from build123d import *

# Parameters (mm, degrees)
CROQUIS1_R                   = 2.5000000000000004
SALIENTE_EXTRUIR1_DEPTH      = 10
SALIENTE_EXTRUIR2_DEPTH      = 12
CROQUIS3_R                   = 1.5000000000000024
SALIENTE_EXTRUIR3_DEPTH      = 2
REDONDEO1_R                  = 2
CROQUIS4_R                   = 1.5000000000000024
CORTAR_EXTRUIR1_DEPTH        = 6
SALIENTE_EXTRUIR4_DEPTH      = 3.21644
SALIENTE_EXTRUIR4_DEPTH_BACK = 18.409513
CROQUIS6_R                   = 2.5
SALIENTE_EXTRUIR5_START      = -21.625954
SALIENTE_EXTRUIR5_DEPTH      = 21.625954


with BuildPart() as part:
    # Croquis1 → Saliente-Extruir1 (new body)
    with BuildSketch(Plane(origin=(0, 0, 0), x_dir=(1, 0, 0), z_dir=(0, 1, 0))):
        with BuildLine():
            Line((0, -4.5), (4.5, -4.5))
            Line((4.5, -4.5), (4.5, 0))
            Line((4.5, 0), (4.5, 4.5))
            Line((4.5, 4.5), (0, 4.5))
            ThreePointArc((0, 4.5), (-4.5, 5.5e-16), (0, -4.5))
        make_face()
        with Locations(Location((0, 0, 0), (0, 0, 270))):
            Circle(CROQUIS1_R, mode=Mode.SUBTRACT)
    extrude(amount=SALIENTE_EXTRUIR1_DEPTH)

    # Croquis2 → Saliente-Extruir2 (add)
    with BuildSketch(Plane(origin=(4.5, 0, 0), x_dir=(0, 0, -1), z_dir=(1, 0, 0))):
        Polygon((-4.5, 0), (-4.5, 1.7434467956210846), (4.5, 14.596778856299984), (4.5, 11.10988526505781), (-3.2792254112385364, 0), align=None)
    extrude(amount=SALIENTE_EXTRUIR2_DEPTH)

    # Croquis3 → Saliente-Extruir3 (add)
    with BuildSketch(Plane(origin=(0, 2.68788483311935, 3.838697366771722), x_dir=(1, 0, 0), z_dir=(0, 0.57357643635105, 0.819152044288989))):
        Polygon((4.5, 19.19256462345726), (16.5, 19.19256462345726), (16.500000000000004, -5.807435376542737), (4.500000000000008, -5.807435376542739), align=None)
        with Locations(Location((10.5, 14.692564623457262, 0), (0, 0, 270))):
            Circle(CROQUIS3_R, mode=Mode.SUBTRACT)
        with Locations((10.500000000000002, -1.307435376542739)):
            Circle(CROQUIS3_R, mode=Mode.SUBTRACT)
    extrude(amount=-SALIENTE_EXTRUIR3_DEPTH)

    # Redondeo1
    # the kernel refuses this fillet: 2 mm, written as the material it adds along each edge
    with BuildSketch(Plane(origin=(4.5, 14.095760221444946, -6.590732152613882), x_dir=(0, -0.5735764363510499, -0.8191520442889891), z_dir=(0, -0.8191520442889891, 0.5735764363510499))) as redondeo1_piece_1_section:
        with BuildLine():
            CenterArc((REDONDEO1_R, REDONDEO1_R), REDONDEO1_R, 180, 90)
            Line((2.9e-16, REDONDEO1_R), (0, 0))
            Line((0, 0), (REDONDEO1_R, 0))
        make_face()
    redondeo1_piece_1 = extrude(amount=22.207745887614607, mode=Mode.PRIVATE)
    redondeo1_piece_1 = split(redondeo1_piece_1, bisect_by=Plane(origin=(4.952132948242019, 4.929093638164552, -4.5), z_dir=(0, 0, 1)), keep=Keep.TOP, mode=Mode.PRIVATE)
    redondeo1_piece_1 = split(redondeo1_piece_1, bisect_by=Plane(origin=(4.952132948242019, 10, -0.7036487498955591), z_dir=(0, -1, 0)), keep=Keep.TOP, mode=Mode.PRIVATE)
    redondeo1_piece_1 = split(redondeo1_piece_1, bisect_by=Plane(origin=(4.952132948242019, 0, -0.7036487498955591), z_dir=(0, 1, 0)), keep=Keep.TOP, mode=Mode.PRIVATE)
    add(redondeo1_piece_1)

    # Croquis4 → Cortar-Extruir1 (cut)
    with BuildSketch(Plane(origin=(0, 2.68788483311935, 3.838697366771722), x_dir=(1, 0, 0), z_dir=(0, 0.57357643635105, 0.819152044288989))):
        with Locations(Location((10.5, 14.69256462345726, 0), (0, 0, 270))):
            Circle(CROQUIS4_R)
        with Locations(Location((10.500000000000002, -1.3074353765427391, 0), (0, 0, 270))):
            Circle(CROQUIS4_R)
    extrude(amount=-CORTAR_EXTRUIR1_DEPTH, mode=Mode.SUBTRACT)

    # Croquis6 → Saliente-Extruir4 (add, two sides: drawn at the far end of the back side and taken through both)
    with BuildSketch(Plane.XZ.offset(-SALIENTE_EXTRUIR4_DEPTH_BACK)):
        with BuildLine():
            Line((4.5, -4.5), (0, -4.5))
            ThreePointArc((0, -4.5), (-4.5, 5.5e-16), (0, 4.5))
            Line((0, 4.5), (4.500000000000005, 4.5))
            Line((4.500000000000005, 4.5), (4.5, -4.5))
        make_face()
        with Locations(Location((0, 0, 0), (0, 0, 270))):
            Circle(CROQUIS6_R, mode=Mode.SUBTRACT)
    extrude(amount=SALIENTE_EXTRUIR4_DEPTH + SALIENTE_EXTRUIR4_DEPTH_BACK)

    # Croquis7 → Saliente-Extruir5 (add)
    with BuildSketch(Plane(origin=(0, 18.409513379572896, 0), x_dir=(1, 0, 0), z_dir=(0, 1, 0)).offset(SALIENTE_EXTRUIR5_START)):
        Polygon((5.5e-16, -4.5), (1.8007390664454916, -7.169705454388125), (4.500000000000005, -7.169705454388125), (4.500000000000005, -4.5), align=None)
    extrude(amount=SALIENTE_EXTRUIR5_DEPTH)


solid = part.part
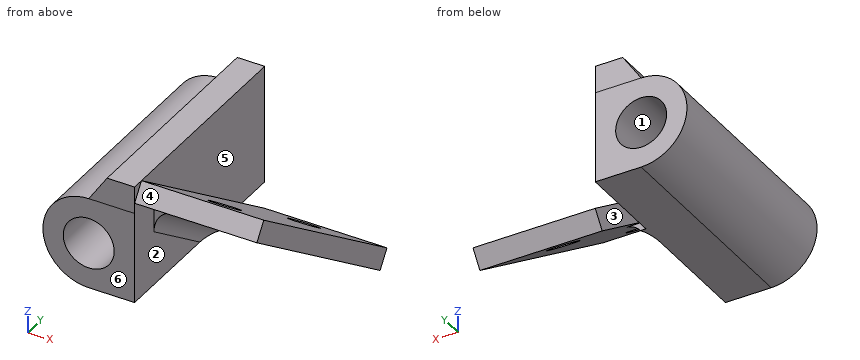
Geometry check sheet. Reference: the model listing, model coordinates, mm. Face numbers are marked on the shaded views. A direction names the side the tool comes from. Coordinates: 2 decimals unless noted, no trailing zeros. Write each loop counter-clockwise with the first axis right and the second up, starting at its lowest first coordinate (ties: lowest second). Pieces come first, ordered by that corner, then holes. Notation, with made-up numbers: (89.5, 36) -> (131.5, 36) arc R20 cw to (131.5, 52) -> close; hole circle Ø6 at (42, -35). An arc over 180 degrees is marked (long way). One line per question, with ' | ' between items.
1. Cross-section at B-B on x = 13.25. Record the cut outline in (y, z).
Answers:
outline: (-3.22, 5.53) -> (17.26, -8.81) -> (18.41, -7.17) -> (-2.07, 7.17) -> close
2. Draft check along X on the marked faces 1, 2, 3 and 4. Enter one of: +X half, -X half, draft (parallel to the pull), parting line (faces both ways), or undercut.
Answers:
face 1: undercut | face 2: +X half | face 3: -X half | face 4: draft
3. Cross-section at A-A on y = 10.5. Record the cut outline in (x, z).
Answers:
outline: (0, -4.5) -> (4.5, -4.5) -> (4.5, -4.07) -> (16.5, -4.07) -> (16.5, -1.63) -> (4.5, -1.63) -> (4.5, 7.17) -> (1.8, 7.17) -> (0, 4.5) arc R4.5 ccw to start; hole circle Ø5 at (0, 0)
4. Depth check by flat-ended pin: pin 1 Ø1.3 at (y, z) = (16, -6) entering from -X; pin 2 Ø4.5 at (x, z) = (0, 0) entering from -Y; pin 3 Ø2 at (x, y) = (8, 11) entering from -Z; pin 4 Ø6 at (x, y) = (11.5, 0) entering from +Z. Enter the tip coordinate at first touch or a pass-through.
Answers:
pin 1: stops at x = 4.5 | pin 2: passes through | pin 3: stops at z = -5.12 | pin 4: stops at z = 7.17
5. Set-up check for the marked faces 5 and 6: record each of +Z, -Z, +X, -X, +Y, -Y from which the full face is reachable in a straight line by a thin tool's end or side.
Answers:
face 5: +Z, +X, +Y | face 6: +Z, -Z, +X, -X, -Y
6. Thickness scan on probe 1 along X at (y, z) = (5, 0); probe 2 along X at (y, z) = (1.5, 0); probe 3 along Z at (x, y) = (4.25, 14.25). Record the ranges inside material, lowest first. Write a range as from..to.
Answers:
probe 1: x = -4.5..-2.5, 2.5..16.5 | probe 2: x = -4.5..-2.5, 2.5..4.51 | probe 3: z = -4.5..7.17
